Study the drawing (mm; zero at the part's minimum x, y, z) and answer. A direction names the side the tool comes from. Give positions to 0.01 mm unless a question says otherwise; leave off trailing zeros. Loops run counter-clockwise (first coordinate to the right, second up) from the corner with the lowest first, then second, coordinate; pieces in that order, holes last. Notation, with made-up numbers: M 78.5,58.5 L 125.5,58.5 A25 ccw 125.5,75.5 Z; hole C 89,-24.75 d2. An arc over 180 degrees is marked long. Return JSON: item names as keys, results as strings.
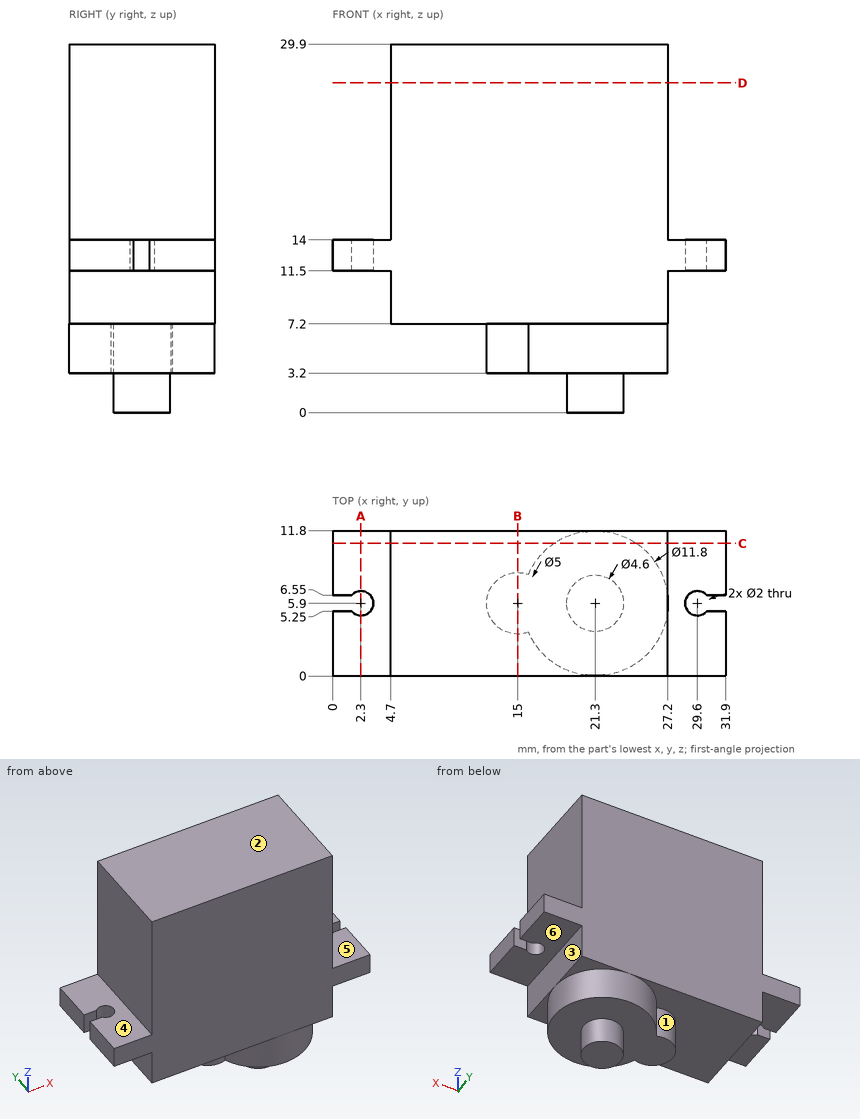
(1) Given pin 1 (2.5 mm diameter, centred on x = 29.6, y = 5.9, fed in from +Z); pin 2 (2.5 mm diameter, centred on x = 30, y = 6.5, fed in from -Z); pin 3 (3.5 mm diameter, centred on y = 8, z = 20, fed in from +X); pin 4 (1.8 mm diameter, centred on x = 2.3, y = 5.9, fed in from +Z), each flat-ended and moving along its own axis, determine where each tip first touches the part or whether it passes through.
Values follow:
{"pin 1": "z = 14", "pin 2": "z = 11.5", "pin 3": "x = 27.2", "pin 4": "through"}
(2) The part is cut by section A-A (x = 2.3). Determine the outline of the cut face in (y, z).
Values follow:
{"outline": "M 0,11.5 L 4.9,11.5 L 4.9,14 L 0,14 Z; M 6.9,11.5 L 11.8,11.5 L 11.8,14 L 6.9,14 Z"}
(3) Straight lines are drawn through the part: line 1 along Y through (x, z) = (29.6, 12.8); line 2 along Z through (x, y) = (13.5, 3); line 3 along X through (y, z) = (5.9, 13.4). For each, find the intervals that lie inside material, in ascending order.
Values follow:
{"line 1": "0 to 4.9, 6.9 to 11.8", "line 2": "7.2 to 29.9", "line 3": "3.3 to 28.6"}
(4) Determine the mould class of the marked faces 1, 2 and 3 for opening direction X: released by +X, released by -X, zero draft, split by the parting line, or undercut.
Values follow:
{"face 1": "undercut", "face 2": "zero draft", "face 3": "released by +X"}
(5) The part is cut by section D-D (z = 26.75). Determine the outline of the cut face in (x, y), and give its area (4 significant figures).
Values follow:
{"outline": "M 4.7,0 L 27.2,0 L 27.2,11.8 L 4.7,11.8 Z", "area": "265.5 mm²"}
(6) A tool of negligible diameter and unlimited length cuts with its end or side. For the marked faces 4, 5 and 6, from which of +Z, -Z, +X, -X, +Y, -Y can it reach the whole face along a straight path? Write none if from no direction.
Values follow:
{"face 4": "+Z, -X, +Y, -Y", "face 5": "+Z, +X, +Y, -Y", "face 6": "-Z, +X, +Y, -Y"}
(7) The part is cut by section B-B (x = 15). Determine the outline of the cut face in (y, z), and give its area (3 significant figures).
Values follow:
{"outline": "M 0,7.2 L 3.4,7.2 L 3.4,3.2 L 8.4,3.2 L 8.4,7.2 L 11.8,7.2 L 11.8,29.9 L 0,29.9 Z", "area": "288 mm²"}
(8) The part is cut by section C-C (y = 10.75). Determine the outline of the cut face in (x, z).
Values follow:
{"outline": "M 0,11.5 L 4.7,11.5 L 4.7,7.2 L 17.94,7.2 L 17.94,3.2 L 24.66,3.2 L 24.66,7.2 L 27.2,7.2 L 27.2,11.5 L 31.9,11.5 L 31.9,14 L 27.2,14 L 27.2,29.9 L 4.7,29.9 L 4.7,14 L 0,14 Z"}
